Read the model definition and answer for the solid it produces. Units are mm, in the model's axes. Round coordinates to 2 decimals unless told otherwise and drop trailing zeros. Order: outer loops, then holes, each group sorted by start corner. A loop starts at its lowest first (then second) coordinate and runs counter-clockwise, first axis right, second up. Notation, with made-up numbers: (32.5, 40.25) -> (58.5, 40.25) arc R11 ccw to (58.5, 46.25) -> close; hole circle Ø8 at (-30, 35.25). An arc over 180 degrees is marked (long way). One line per item, written item: value. Start each with the question number.
1. Section D-D (x = -31) is taken. Give the vertices of the cut face in (y, z).
2. Section C-C (x = 36) is taken. Give the vertices of the cut face in (y, z).
3. Section A-A (y = -27.5) is taken. Give the vertices of the cut face in (x, z), then the cut area to 3 significant figures.
4. Section B-B (z = 0.75) is taken. State how many separate pieces and enclosed holes the cut face has, then the cut area to 3 significant figures.
5. Flat-ended cylindrical pins translate along their axes: pin 1 Ø2.5 at (x, y) = (-25.5, 7.5) entering from +Z; pin 2 Ø1.9 at (x, y) = (-36, 20) entering from +Z. Find the tip coordinate at first contact, or state that the pin passes through.
6. Consider line 1 (X direction, y = 7.5, z = 0.3); line 2 (X direction, y = 20, z = 0.65); line 3 (Y direction, x = -25.5, z = 0.95). Determine where each line is inside the solid, lowest interval first.
Autodesk Inventor part; units mm, degrees
ref_plane "YZ Plane" through (0, 0, 0) normal (1, 0, 0) x (0, 1, 0)
ref_plane "XZ Plane" through (0, 0, 0) normal (0, 1, 0) x (-1, 0, 0)
ref_plane "XY Plane" through (0, 0, 0) normal (0, 0, 1) x (1, 0, 0)
sketch "スケッチ1" plane through (0, 0, 0) normal (0, 0, 1) x (1, 0, 0)
  circle A0 centre (0, 0) radius 60 construction
  line L0 (-40, 60) -> (40, 60) construction
  line L1 (40, 60) -> (40, -60) construction
  line L2 (40, -60) -> (-40, -60) construction
  line L3 (-40, -60) -> (-40, 60) construction
  arc A1 (40, 44.7214) -> (-40, 44.7214) centre (0, 0) ccw
  line L4 (-40, 44.7214) -> (-40, -44.7214)
  line L5 (40, 44.7214) -> (40, -44.7214)
  arc A2 (-40, -44.7214) -> (40, -44.7214) centre (0, 0) ccw
  line L6 (40, -44) -> (-40, -44)
  point P0 (0, 60)
  dimension "d0" = 120
  dimension "d1" = 80
  dimension "d41" = 44
extrude "基板" add sketch "スケッチ1" along normal blind 1.6 contours L5 L6 L4 A1
sketch "スケッチ2" plane through (0, 0, 1.6) normal (0, 0, 1) x (1, 0, 0)
  line L0 (0, 110.7931) -> (0, -110.7931) construction
  line L1 (-40, 44.7214) -> (-40, -44) construction
  line L2 (-63.4163, -10) -> (63.4163, -10) construction
  point P0 (0, 0)
  point P1 (0, 0)
  point P2 (0, 0)
  point P3 (-42.5, -49.1808)
  point P4 (-25.5, -27.5)
  point P5 (-25.5, 7.5)
  point P6 (25.5, -27.5)
  point P7 (25.5, 7.5)
  point P8 (0, -10)
  point P9 (-40, -44)
  dimension "BLACKET_SPAN" = 35
  dimension "d40" = 10
  dimension "BLACKET_W" = 51
hole "モータ取付穴" at (-25.5, -27.5, 1.6) at (-25.5, 7.5, 1.6) at (25.5, -27.5, 1.6) at (25.5, 7.5, 1.6) direction (0, 0, -1) diameter 2.1 end through all
sketch "スケッチ6" plane through (0, 0, 0) normal (0, 0, -1) x (-1, 0, 0)
  line L0 (0, 0) -> (0, 96.2051) construction
  point P0 (36, 43)
  point P1 (-36, 43)
  point P2 (-36, 20)
  point P3 (36, 20)
  dimension "CONN_W" = 72
  dimension "CONN_SPAN" = 23
  dimension "CONN_L1" = 43
hole "連結穴" at (-36, 43, 0) at (36, 43, 0) at (36, 20, 0) at (-36, 20, 0) direction (0, 0, 1) diameter 3.2 end through all
properties part number "BaseBoard-SPG27"
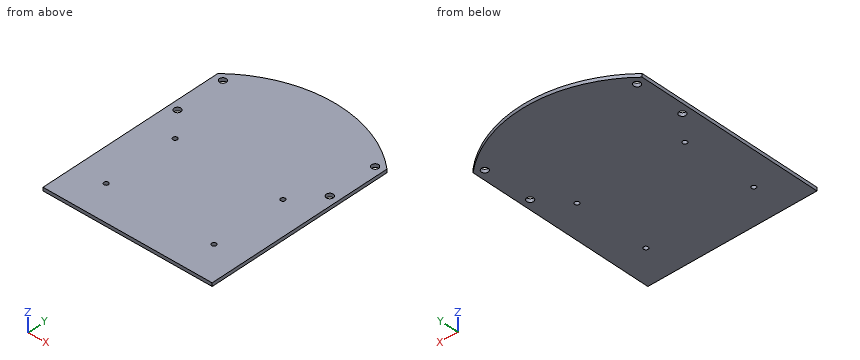
Answer:
1. outline: (-44, 0) -> (51.37, 0) -> (51.37, 1.6) -> (-44, 1.6) -> close
2. outline: (-44, 0) -> (18.4, 0) -> (18.4, 1.6) -> (-44, 1.6) -> close; (21.6, 0) -> (41.4, 0) -> (41.4, 1.6) -> (21.6, 1.6) -> close; (44.6, 0) -> (48, 0) -> (48, 1.6) -> (44.6, 1.6) -> close
3. outline: (-40, 0) -> (-26.55, 0) -> (-26.55, 1.6) -> (-40, 1.6) -> close; (-24.45, 0) -> (24.45, 0) -> (24.45, 1.6) -> (-24.45, 1.6) -> close; (26.55, 0) -> (40, 0) -> (40, 1.6) -> (26.55, 1.6) -> close
3. area: 121 mm^2
4. separate pieces: 1
4. enclosed holes: 8
4. area: 7,890 mm^2
5. pin 1: z = 1.6
5. pin 2: through
6. line 1: -40 to -26.55, -24.45 to 24.45, 26.55 to 40
6. line 2: -40 to -37.6, -34.4 to 34.4, 37.6 to 40
6. line 3: -44 to -28.55, -26.45 to 6.45, 8.55 to 54.31
